Geometry check sheet. Reference: the model listing, model coordinates, mm. Give positions to 0.01 mm unless a question says otherwise; leave off trailing zeros. Loops run counter-clockwise (first coordinate to the right, second up) from the corner with the lowest first, then second, coordinate; pieces in that order, holes last. Notation, with made-up numbers: (-2, 23) -> (11, 23) arc R14 ccw to (11, 41) -> close; hole circle Ø8 at (-13.75, 45). An arc over 180 degrees is marked (long way). Write item = value, one per line. Start each with the question number.
```python
from build123d import *

# Parameters (mm, degrees)
EXTRUDE_1_DEPTH  = 25
HOLE_WIZARD_M8_D = 6.8


with BuildPart() as part:
    # Эскиз1 → Бобышка-Вытянуть1 (new body)
    with BuildSketch(Plane.XY):
        Polygon((6.92820323, 0), (3.464101615, 6), (-3.464101615, 6), (-6.92820323, 0), (-3.464101615, -6), (3.464101615, -6), align=None)
    extrude(amount=-EXTRUDE_1_DEPTH)

    # M8 (through all)
    with Locations(Plane.XY):
        with Locations((0, 0)):
            Hole(HOLE_WIZARD_M8_D / 2)


solid = part.part
```
1) Thickness scan on line 1 (Y direction, x = 0, z = -13); line 2 (X direction, y = 2.25, z = -16.75); line 3 (Y direction, x = 2, z = -22). Record the ranges inside material, lowest first.
2) Section check B-B (z = -11). Enter the section's corners in (x, y), plus the area to 3 significant figures.
3) Section check D-D (x = -5.5). Enter the section's corners in (y, z).
4) Section check C-C (y = 2). Enter the section's corners in (x, z).
5) Section check A-A (x = 0). Enter the section's corners in (y, z).
6) Draft check along X on faces 1 (the flat face through (0, 6, -12)), 2 (the cylindrical face through (0.74, -3.32, -12.68)), 3 (the flat face through (5.22, 2.96, -12.32)). Enter one of: released by +X, released by -X, zero draft, split by the parting line, or undercut.
7) Depth check by flat-ended pin: pin 1 Ø5 at (y, z) = (4, -4) entering from +X; pin 2 Ø3 at (y, z) = (1, -20.5) entering from -X; pin 3 Ø4 at (y, z) = (-4.5, -11) entering from -X; pin 4 Ø5.5 at (x, y) = (0, 0) entering from +Z. Enter the tip coordinate at first touch or a pass-through.
Check result:
q1.line_1 = -6 to -3.4, 3.4 to 6
q1.line_2 = -5.63 to -2.55, 2.55 to 5.63
q1.line_3 = -6 to -2.75, 2.75 to 6
q2.outline = (-6.93, 0) -> (-3.46, -6) -> (3.46, -6) -> (6.93, 0) -> (3.46, 6) -> (-3.46, 6) -> close; hole circle Ø6.8 at (0, 0)
q2.area = 88.4 mm2
q3.outline = (-2.47, -25) -> (2.47, -25) -> (2.47, 0) -> (-2.47, 0) -> close
q4.outline = (-5.77, -25) -> (-2.75, -25) -> (-2.75, 0) -> (-5.77, 0) -> close; (2.75, -25) -> (5.77, -25) -> (5.77, 0) -> (2.75, 0) -> close
q5.outline = (-6, -25) -> (-3.4, -25) -> (-3.4, 0) -> (-6, 0) -> close; (3.4, -25) -> (6, -25) -> (6, 0) -> (3.4, 0) -> close
q6.face_1 = zero draft
q6.face_2 = undercut
q6.face_3 = released by +X
q7.pin_1 = 6.06
q7.pin_2 = -6.93
q7.pin_3 = -5.48
q7.pin_4 = through
